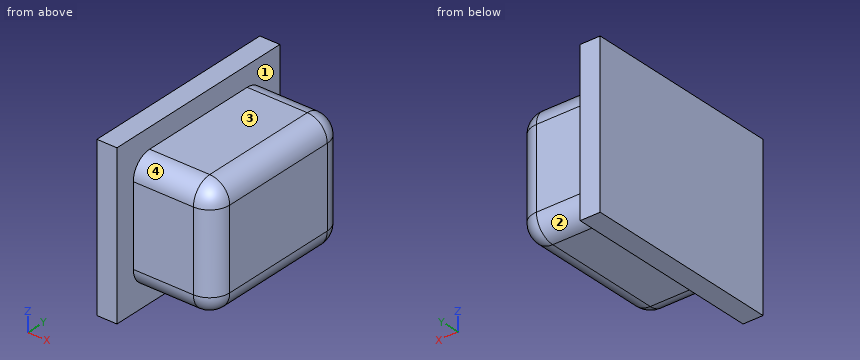
Autodesk Inventor part; units mm, degrees
ref_plane "YZ Plane" through (0, 0, 0) normal (1, 0, 0) x (0, 1, 0)
ref_plane "XZ Plane" through (0, 0, 0) normal (0, 1, 0) x (-1, 0, 0)
ref_plane "XY Plane" through (0, 0, 0) normal (0, 0, 1) x (1, 0, 0)
sketch "Sketch1" plane through (0, 0, 0) normal (1, 0, 0) x (0, 1, 0)
  line L0 (0, 0) -> (12.6492, 0)
  line L1 (12.6492, 0) -> (12.6492, -9.4742)
  line L2 (12.6492, -9.4742) -> (0, -9.4742)
  line L3 (0, -9.4742) -> (0, 0)
  dimension "d0" = 12.6492
  dimension "d1" = 9.4742
extrude "Extrusion1" add sketch "Sketch1" along normal mid plane 6.35
sketch "Sketch2" plane through (-3.175, 0, 0) normal (-1, 0, 0) x (0, 0, 1)
  line L0 (0, 0) -> (0, 12.6492)
  line L1 (0, 12.6492) -> (-9.4742, 12.6492)
  line L2 (-9.4742, 12.6492) -> (-9.4742, 0)
  line L3 (-9.4742, 0) -> (0, 0)
  line L4 (1.5875, 14.2367) -> (1.5875, -1.5875)
  line L5 (1.5875, -1.5875) -> (-11.0617, -1.5875)
  line L6 (-11.0617, -1.5875) -> (-11.0617, 14.2367)
  line L7 (-11.0617, 14.2367) -> (1.5875, 14.2367)
  dimension "d4" = 1.5875
extrude "Extrusion2" add sketch "Sketch2" along normal blind 1.5875 contours L3 L2 L1 L0 | L4 L5 L6 L7
fillet "Fillet1" radius 1.5875 8 edges at (0, 12.6492, 0) (3.175, 12.6492, -4.7371) (0, 12.6492, -9.4742) (3.175, 6.3246, -9.4742) (0, 0, -9.4742) (3.175, 0, -4.7371) (0, 0, 0) (3.175, 6.3246, 0)
properties part number "Button" material "ABS Plastic"
Check sheet for the modelled part. Datum: model origin and axes. Units: mm. Face numbers are marked on the shaded views. A direction names the side the tool comes from. Round coordinates to 2 decimals unless told otherwise and drop trailing zeros. Order: outer loops, then holes, each group sorted by start corner. A loop starts at its lowest first (then second) coordinate and runs counter-clockwise, first axis right, second up.
1) Section check A-A (z = -6). Record the boundary of the cut face in (x, y) (1 decimal), and give its area (3 significant figures).
2) Go/stop test with flat-tipped pins: pin 1 Ø1 at (x, z) = (-2, -2) entering from +Y; pin 2 Ø1 at (x, y) = (0.5, 4.5) entering from +Z; pin 3 Ø2.5 at (x, y) = (-0.5, 4) entering from -Z. Record where each tip stops, or that it passes through.
3) Section check B-B (y = 3.5). Record the boundary of the cut face in (x, z) (1 decimal), and give its area (3 significant figures).
4) Section check C-C (x = -3). Record the boundary of the cut face in (y, z) (1 decimal), and give its area (3 significant figures).
5) Scan lines: line 1 (Y direction, x = 0, z = -7.5); line 2 (Z direction, x = 1.5, y = 7.75); line 3 (X direction, y = -0.5, z = -9.75) (1 decimal). Record each from-to range of solid material in increasing order.
6) Tool access check on the marked faces 1, 2, 3 and 4. Record the directions out of +Z, -Z, +X, -X, +Y, -Y that give a thin tool (end or side, any length) a straight path to the whole face; none if there is none.
Result:
1. outline: (-4.8, -1.6) - (-3.2, -1.6) - (-3.2, 0) - (1.6, 0) arc R1.6 ccw to (3.2, 1.6) - (3.2, 11.1) arc R1.6 ccw to (1.6, 12.6) - (-3.2, 12.6) - (-3.2, 14.2) - (-4.8, 14.2) - close
1. area: 104 mm2
2. pin 1: stops at y = 12.65
2. pin 2: stops at z = 0
2. pin 3: stops at z = -9.47
3. outline: (-4.8, -11.1) - (-3.2, -11.1) - (-3.2, -9.5) - (1.6, -9.5) arc R1.6 ccw to (3.2, -7.9) - (3.2, -1.6) arc R1.6 ccw to (1.6, 0) - (-3.2, 0) - (-3.2, 1.6) - (-4.8, 1.6) - close
3. area: 79.2 mm2
4. outline: (0, -7.9) arc R1.6 ccw to (1.6, -9.5) - (11.1, -9.5) arc R1.6 ccw to (12.6, -7.9) - (12.6, -1.6) arc R1.6 ccw to (11.1, 0) - (1.6, 0) arc R1.6 ccw to (0, -1.6) - close
4. area: 118 mm2
5. line 1: y = 0 to 12.65
5. line 2: z = -9.47 to 0
5. line 3: x = -4.8 to -3.2
6. face 1: +X
6. face 2: -Z, +X, +Y
6. face 3: +Z, +X, +Y, -Y
6. face 4: +Z, +X, -Y
